Here's how the part is built. I have some questions about the finished solid (model axes, mm). A direction names the side the tool comes from. Round coordinates to 2 decimals unless told otherwise and drop trailing zeros. Order: outer loops, then holes, each group sorted by start corner. A loop starts at its lowest first (then second) coordinate and runs counter-clockwise, first axis right, second up. Notation, with made-up numbers: (79, -8.75) - (94, -8.75) arc R8 ccw to (94, 3.25) - close; hole circle Ø6 at (31.5, -5). An arc over 180 degrees is marked (long way). Answer as a JSON object with one key per item and string values.
```python
from build123d import *

# Parameters (mm, degrees)
CROQUIS3_W              = 790
CROQUIS3_H              = 790
SALIENTE_EXTRUIR1_DEPTH = 210
VACIADO2_T              = -0.76
CROQUIS5_W              = 160
CROQUIS5_H              = 160
CROQUIS5_W_2            = 158.245179758
CROQUIS5_H_2            = 158.245179758
SALIENTE_EXTRUIR2_DEPTH = 40


with BuildPart() as part:
    # Croquis1 → Recubrir1 section 0
    with BuildSketch(Plane(origin=(0, 0, 0), x_dir=(1, 0, 0), z_dir=(0, 1, 0))):
        with BuildLine():
            Line((-395, 395), (395, 395))
            Line((395, 395), (395, -395))
            Line((395, -395), (-395, -395))
            Line((-395, -395), (-395, 395))
        make_face()
    # Croquis2 → Recubrir1 section 1
    with BuildSketch(Plane(origin=(0, -546, 0), x_dir=(1, 0, 0), z_dir=(0, 1, 0))):
        with BuildLine():
            Line((-80, 80), (80, 80))
            Line((80, 80), (80, -80))
            Line((80, -80), (-80, -80))
            Line((-80, -80), (-80, 80))
        make_face()
    loft()

    # Croquis3 → Saliente-Extruir1 (add)
    with BuildSketch(Plane(origin=(0, 0, 0), x_dir=(1, 0, 0), z_dir=(0, 1, 0))):
        Rectangle(CROQUIS3_W, CROQUIS3_H)
    extrude(amount=SALIENTE_EXTRUIR1_DEPTH)

    # Vaciado2
    vaciado2_openings = [part.faces().sort_by_distance(p)[0] for p in [
        (0, -546, 0),
        (0, 210, 0),
    ]]
    offset(amount=VACIADO2_T, openings=vaciado2_openings)

    # Croquis5 → Saliente-Extruir2 (add)
    with BuildSketch(Plane.XZ.offset(546)):
        Rectangle(CROQUIS5_W, CROQUIS5_H)
        Rectangle(CROQUIS5_W_2, CROQUIS5_H_2, mode=Mode.SUBTRACT)
    extrude(amount=SALIENTE_EXTRUIR2_DEPTH)


solid = part.part
```
1. Imagine slicing it at A-A (y = 42.5). List the corners of the cut face in (x, z) for me, plus the area to 3 significant figures.
Responses:
{"outline": "(-395, -395) - (395, -395) - (395, 395) - (-395, 395) - close; hole (-394.24, -394.24) - (394.24, -394.24) - (394.24, 394.24) - (-394.24, 394.24) - close", "area": "2,400 mm2"}
2. Thinking about a two-plate mould opening in Z: for faces 6 (the face through (-6, 104, 394.24)), 7 (the face through (-1, -566, 80)), 8 (the face through (-6, 104, -394.24)), 9 (the face through (-1, -566, -80)), which applies, pulls with the +Z half, pulls with the -Z half, needs draft (parallel to the pull), parting line crosses it, or undercut?
Responses:
{"face 6": "undercut", "face 7": "pulls with the +Z half", "face 8": "undercut", "face 9": "pulls with the -Z half"}
3. For P1, Ø12, axis at y = -564, z = -6.5, coming from the +X side; P2, Ø12, axis at y = -560, z = -37.5, coming from the -X side; P3, Ø12, axis at x = -27, y = -556, coming from the -Z side, each with a flat end and sliding along its axis, tell me the tip position at first contact or that it passes through.
Responses:
{"P1": "x = 80", "P2": "x = -80", "P3": "z = -80"}
4. For faces 1 (the face through (79.123, -566, -1)), 2 (the face through (-80, -566, -1)), 3 (the face through (80, -566, -1)), 4 (the face through (394.24, 104, 6)), 5 (the face through (-395, 104, 6)), which set-ups out of +Z, -Z, +X, -X, +Y, -Y let a thin tool reach every point of the face, with its end or its side?
Responses:
{"face 1": "+Y, -Y", "face 2": "+Z, -Z, -X, -Y", "face 3": "+Z, -Z, +X, -Y", "face 4": "+Y", "face 5": "+Z, -Z, -X, +Y, -Y"}
5. If I drill on L1, parallel to X at y = 52, z = 106.5; L2, parallel to Z at x = -86, y = -160.5, over which ranges is the centre line in solid material (lowest first)? Write a range as [from, to].
Responses:
{"L1": "[-395, -394.24], [394.24, 395]", "L2": "[-302.4, -301.53], [301.53, 302.4]"}
